Here's how the part is built. I have some questions about the finished solid (model axes, mm). Round coordinates to 2 decimals unless told otherwise and drop trailing zeros. Loops run counter-clockwise (first coordinate to the right, second up) from the corner with the lowest first, then second, coordinate; pieces in that order, holes last. Notation, with made-up numbers: (65.25, 17) - (92.25, 17) arc R6 ccw to (92.25, 26) - close; hole circle Ø9 at (-14.75, 89). An arc over 180 degrees is marked (long way). Return JSON: item names as keys, results as strings. Group by question number.
Autodesk Inventor part; units mm, degrees
ref_plane "YZ Plane" through (0, 0, 0) normal (1, 0, 0) x (0, 1, 0)
ref_plane "XZ Plane" through (0, 0, 0) normal (0, 1, 0) x (-1, 0, 0)
ref_plane "XY Plane" through (0, 0, 0) normal (0, 0, 1) x (1, 0, 0)
sketch "Эскиз1" plane through (0, 0, 0) normal (0, 1, 0) x (-1, 0, 0)
  circle A0 centre (0, 0) radius 22
  dimension "d0" = 44
extrude "Выдавливание1" add sketch "Эскиз1" against normal blind 3
sketch "Эскиз2" plane through (0, -3, 0) normal (0, -1, 0) x (1, 0, 0)
  circle A0 centre (0, 0) radius 4.25
  dimension "d3" = 8.5
extrude "Выдавливание2" add sketch "Эскиз2" along normal blind 2
sketch "Эскиз3" plane through (0, -5, 0) normal (0, -1, 0) x (1, 0, 0)
  circle A0 centre (0, 0) radius 1.5
  dimension "d6" = 3
extrude "Выдавливание3" cut sketch "Эскиз3" against normal through all
equation "\"d0\" = 14.6667 * d6"
equation "\"d3\" = 2.83333 * d6"
properties material "Медь, ковкая"
Q1. Imagine slicing it at D-D, the plane z = -14.5. List the corners of the cut face in (x, y) for me.
Q2. Imagine slicing it at B-B, the plane z = 1. List the corners of the cut face in (x, y) for me, and give its area (3 significant figures).
Q3. Imagine slicing it at C-C, the plane y = -1.2. List the corners of the cut face in (x, z) for me, and give its area (3 significant figures).
Q4. Please list where these lines run through material, in increasing order: line 1 (Z direction, x = 0, y = -1.05); line 2 (Y direction, x = 10.5, z = -11); line 3 (X direction, y = -2.5, z = -10).
Q5. If we mould it in two halves opening along Z, with no side actions, what happens to faces 1 (the cylindrical face through (2.285, -3.986, -3.584)), 2 (the flat face through (2, -5, 0)), 3 (the cylindrical face through (-1.5, -2.54, 0.07))? For each: +Z half, -Z half, draft (parallel to the pull), parting line (faces both ways), or undercut.
Q6. Imagine slicing it at A-A, the plane x = 0. List the corners of the cut face in (y, z) for me, and give its area (3 significant figures).
Q7. Will these pins go through, and if not, where does the flat tip stop? pin 1 Ø3 at (x, y) = (17.5, -0.5) entering from +Z; pin 2 Ø1.8 at (x, z) = (0, 0) entering from -Y; pin 3 Ø1.5 at (x, y) = (7, -1) entering from +Z; pin 4 Ø3 at (y, z) = (-4, -5.5) entering from +X.
Output values:
{
 "1": {"outline": "(-16.55, -3) - (16.55, -3) - (16.55, 0) - (-16.55, 0) - close"},
 "2": {"outline": "(-21.98, -3) - (-4.13, -3) - (-4.13, -5) - (-1.12, -5) - (-1.12, 0) - (-21.98, 0) - close; (1.12, -5) - (4.13, -5) - (4.13, -3) - (21.98, -3) - (21.98, 0) - (1.12, 0) - close", "area": "137 mm^2"},
 "3": {"outline": "circle Ø44 at (0, 0); hole circle Ø3 at (0, 0)", "area": "1,510 mm^2"},
 "4": {"line 1": "z = -22 to -1.5, 1.5 to 22", "line 2": "y = -3 to 0", "line 3": "x = -19.6 to 19.6"},
 "5": {"face 1": "parting line", "face 2": "draft", "face 3": "undercut"},
 "6": {"outline": "(-5, -4.25) - (-3, -4.25) - (-3, -22) - (0, -22) - (0, -1.5) - (-5, -1.5) - close; (-5, 1.5) - (0, 1.5) - (0, 22) - (-3, 22) - (-3, 4.25) - (-5, 4.25) - close", "area": "134 mm^2"},
 "7": {"pin 1": "stops at z = 15.1", "pin 2": "passes through", "pin 3": "stops at z = 21.09", "pin 4": "stops at x = 21.56"}
}
